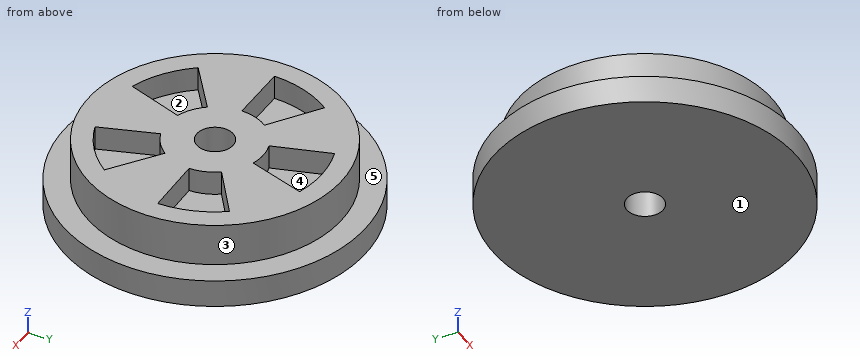
```python
from build123d import *

# Parameters (mm, degrees)
F0_R     = 3.175
F1_DEPTH = 0.5842
F2_R     = 2.667
F3_DEPTH = 0.89916
F4_R     = 0.381
F5_DEPTH = 25.4
F7_DEPTH = 0.508


with BuildPart() as f1:
    # F0 (on Top) → F1 (new body)
    with BuildSketch(Plane.XY):
        Circle(F0_R)
    extrude(amount=F1_DEPTH)

    # F2 (on face) → F3 (join)
    with BuildSketch(Plane.XY.offset(0.5842)):
        Circle(F2_R)
    extrude(amount=F3_DEPTH)

    # F4 (on face) → F5 (cut)
    with BuildSketch(Plane.XY.offset(1.48336)):
        Circle(F4_R)
    extrude(amount=-F5_DEPTH, mode=Mode.SUBTRACT)

    # F6 (on face) → F7 (cut)
    with BuildSketch(Plane.XY.offset(1.48336)):
        with BuildLine():
            ThreePointArc((-0.303926, 0.968739), (0, 1.015296), (0.303926, 0.968739))
            Line((0.303926, 0.968739), (0.672974, 2.145047))
            ThreePointArc((0.672974, 2.145047), (0, 2.248137), (-0.672974, 2.145047))
            Line((-0.672974, 2.145047), (-0.303926, 0.968739))
        make_face()
        with BuildLine():
            Line((-0.827407, 0.588408), (-1.832101, 1.302892))
            ThreePointArc((-1.832101, 1.302892), (-2.138105, 0.694713), (-2.248021, 0.02282))
            Line((-2.248021, 0.02282), (-1.015244, 0.010306))
            ThreePointArc((-1.015244, 0.010306), (-0.965604, 0.313744), (-0.827407, 0.588408))
        make_face()
        with BuildLine():
            Line((-0.815292, -0.605083), (-1.805274, -1.339815))
            ThreePointArc((-1.805274, -1.339815), (-1.321422, -1.818781), (-0.71638, -2.130944))
            Line((-0.71638, -2.130944), (-0.323529, -0.962369))
            ThreePointArc((-0.323529, -0.962369), (-0.596776, -0.821392), (-0.815292, -0.605083))
        make_face()
        with BuildLine():
            Line((0.323529, -0.962369), (0.71638, -2.130944))
            ThreePointArc((0.71638, -2.130944), (1.321422, -1.818781), (1.805274, -1.339815))
            Line((1.805274, -1.339815), (0.815292, -0.605083))
            ThreePointArc((0.815292, -0.605083), (0.596776, -0.821392), (0.323529, -0.962369))
        make_face()
        with BuildLine():
            Line((1.015244, 0.010306), (2.248021, 0.02282))
            ThreePointArc((2.248021, 0.02282), (2.138105, 0.694713), (1.832101, 1.302892))
            Line((1.832101, 1.302892), (0.827407, 0.588408))
            ThreePointArc((0.827407, 0.588408), (0.965604, 0.313744), (1.015244, 0.010306))
        make_face()
    extrude(amount=-F7_DEPTH, mode=Mode.SUBTRACT)


solid = f1.part
```
Part model, mm, in its own coordinate system. Face numbers are marked on the shaded views. A direction names the side the tool comes from. Round coordinates to 2 decimals unless told otherwise and drop trailing zeros. Loops run counter-clockwise (first coordinate to the right, second up) from the corner with the lowest first, then second, coordinate; pieces in that order, holes last. Notation, with made-up numbers: (-31.5, 22.25) -> (24.5, 22.25) arc R13 ccw to (24.5, 29.25) -> close; hole circle Ø9 at (83.25, 47). An arc over 180 degrees is marked (long way). Use CSV: the item, a comma, the result in double quotes. Start each with the question number.
1) Cut at C-C, the plane y = -0.25. Write the cut outline in (x, z).
2) Cut at B-B, the plane z = 1.1. Write the cut outline in (x, y).
3) Drop a flat-ended pin along its axis: P1, Ø0.7, axis at x = 1, y = -1.5, coming from the +Z side. Give the stop position or say it passes through.
4) Which spindle directions (+Z, -Z, +X, -X, +Y, -Y) get a long thin tool onto all of the face, cutting with end or side? Do the marked faces 1 and 2. Say none if no direction does.
5) Wall check: L1, parallel to Y at x = 0, z = 0.55 (3 decimals); L2, parallel to Y at x = 0, z = 1.15; L3, parallel to Y at x = -0.25, z = 1.15. Give the ranges that are in metal, low to high. Write a range as [from, to].
6) Pull direction Y, two halves, no side cores. Call the marked faces 3, 4 and 5: +Y half, -Y half, draft (parallel to the pull), parting line (faces both ways), or undercut.
7) Cut at D-D, the plane z = 0.7. Write the cut outline in (x, y).
8) Cut at A-A, the plane x = 0. Write the cut outline in (y, z) (3 decimals), plus the area to 3 significant figures.
Determined:
1,outline,"(-3.17, 0) -> (-0.29, 0) -> (-0.29, 1.48) -> (-2.66, 1.48) -> (-2.66, 0.58) -> (-3.17, 0.58) -> close; (0.29, 0) -> (3.17, 0) -> (3.17, 0.58) -> (2.66, 0.58) -> (2.66, 1.48) -> (0.29, 1.48) -> close"
2,outline,"circle Ø5.33 at (0, 0); hole (-2.25, 0.02) -> (-1.02, 0.01) arc R1.02 cw to (-0.83, 0.59) -> (-1.83, 1.3) arc R2.25 ccw to start; hole (-1.81, -1.34) arc R2.25 ccw to (-0.72, -2.13) -> (-0.32, -0.96) arc R1.02 cw to (-0.82, -0.61) -> close; hole (-0.67, 2.15) -> (-0.3, 0.97) arc R1.02 cw to (0.3, 0.97) -> (0.67, 2.15) arc R2.25 ccw to start; hole circle Ø0.76 at (0, 0); hole (0.32, -0.96) -> (0.72, -2.13) arc R2.25 ccw to (1.81, -1.34) -> (0.82, -0.61) arc R1.02 cw to start; hole (0.83, 0.59) arc R1.02 cw to (1.02, 0.01) -> (2.25, 0.02) arc R2.25 ccw to (1.83, 1.3) -> close"
3,P1,"stops at z = 0.98"
4,face 1,"-Z, +X, -X, +Y, -Y"
4,face 2,"+Z"
5,L1,"y = [-3.175, -0.381], [0.381, 3.175]"
5,L2,"y = [-2.67, -0.38], [0.38, 1.02], [2.25, 2.67]"
5,L3,"y = [-2.66, -0.29], [0.29, 0.98], [2.23, 2.66]"
6,face 3,"parting line"
6,face 4,"undercut"
6,face 5,"draft"
7,outline,"circle Ø5.33 at (0, 0); hole circle Ø0.76 at (0, 0)"
8,outline,"(-3.175, 0) -> (-0.381, 0) -> (-0.381, 1.483) -> (-2.667, 1.483) -> (-2.667, 0.584) -> (-3.175, 0.584) -> close; (0.381, 0) -> (3.175, 0) -> (3.175, 0.584) -> (2.667, 0.584) -> (2.667, 1.483) -> (2.248, 1.483) -> (2.248, 0.975) -> (1.015, 0.975) -> (1.015, 1.483) -> (0.381, 1.483) -> close"
8,area,"6.75 mm2"
